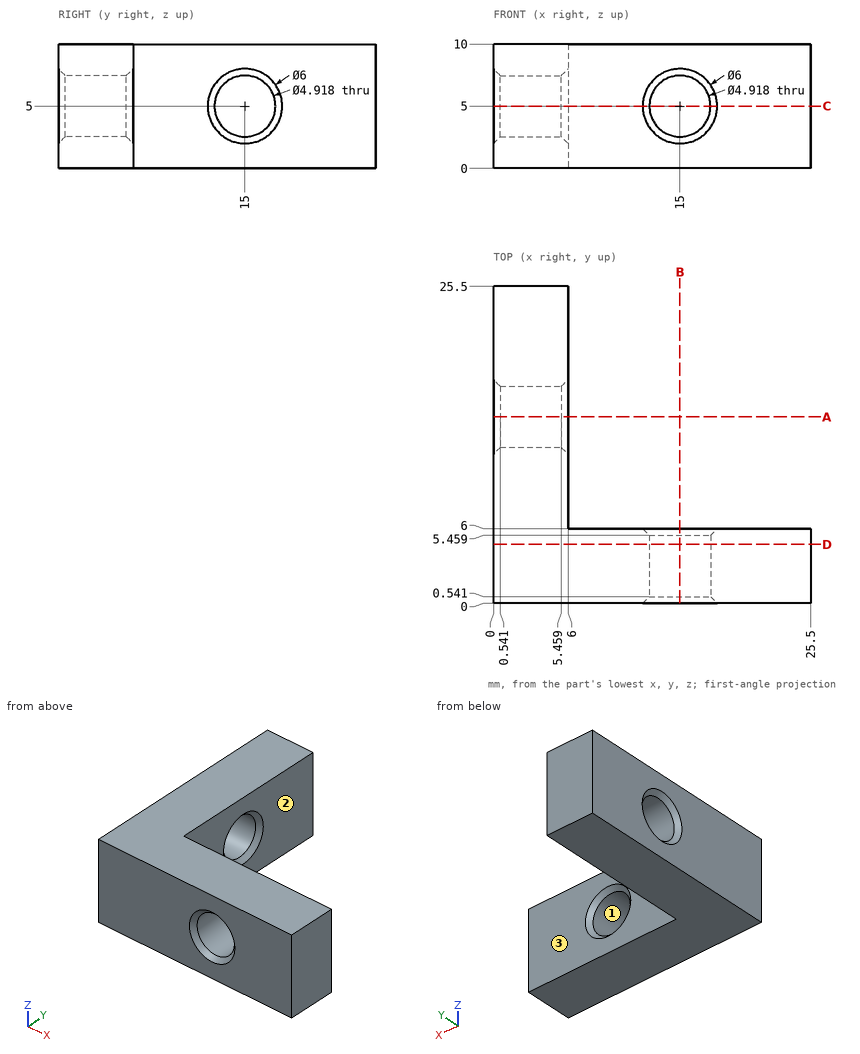
Input: dimensioned drawing with shaded views. Units: mm. Origin: part minimum x, y, z. Give positions to 0.01 mm unless a question says otherwise; leave off trailing zeros. Loops run counter-clockwise (first coordinate to the right, second up) from the corner with the lowest first, then second, coordinate; pieces in that order, holes last. Notation, with made-up numbers: (-33.5, -18) -> (15.5, -18) arc R30 ccw to (15.5, 8) -> close; hole circle Ø10 at (13.25, 86). An arc over 180 degrees is marked (long way). Return JSON: item names as keys, results as strings.
Item 1: Mould query, pull axis X, two halves, no side actions, for the marked faces 1, 2 and 3. Classes: released by +X, released by -X, zero draft, split by the parting line, or undercut.
Filled in:
{"face 1": "undercut", "face 2": "released by +X", "face 3": "zero draft"}
Item 2: Section C-C, the plane z = 5. Output: boundary loops of the cut face in (x, y), plus the area to 3 significant figures.
Filled in:
{"outline": "(0, 0) -> (12, 0) -> (12.54, 0.54) -> (12.54, 5.46) -> (12, 6) -> (6, 6) -> (6, 12) -> (5.46, 12.54) -> (0.54, 12.54) -> (0, 12) -> close; (0, 18) -> (0.54, 17.46) -> (5.46, 17.46) -> (6, 18) -> (6, 25.5) -> (0, 25.5) -> close; (17.46, 0.54) -> (18, 0) -> (25.5, 0) -> (25.5, 6) -> (18, 6) -> (17.46, 5.46) -> close", "area": "210 mm^2"}
Item 3: Line query: line 1 (Y direction, x = 3.65, z = 5); line 2 (Z direction, x = 15, y = 3.2). Output: solid intervals per line, ascending.
Filled in:
{"line 1": "0 to 12.54, 17.46 to 25.5", "line 2": "0 to 2.54, 7.46 to 10"}
Item 4: Pin query (flat end, axial travel): P1, Ø2, axis at x = 13, z = 6.5, coming from the -Y side; P2, Ø3, axis at y = 11, z = 6.5, coming from the +X side. Return the tip coordinate at first contact, or that it passes through.
Filled in:
{"P1": "y = 0", "P2": "x = 6"}
Item 5: Section A-A, the plane y = 15. Output: boundary loops of the cut face in (x, z).
Filled in:
{"outline": "(0, 0) -> (6, 0) -> (6, 2) -> (5.46, 2.54) -> (0.54, 2.54) -> (0, 2) -> close; (0, 8) -> (0.54, 7.46) -> (5.46, 7.46) -> (6, 8) -> (6, 10) -> (0, 10) -> close"}
Item 6: Section D-D, the plane y = 4.75. Output: boundary loops of the cut face in (x, z).
Filled in:
{"outline": "(0, 0) -> (25.5, 0) -> (25.5, 10) -> (0, 10) -> close; hole circle Ø4.92 at (15, 5)"}
